Here's how the part is built. I have some questions about the finished solid (model axes, mm). Give positions to 0.01 mm unless a question says otherwise; leave off trailing zeros. Loops run counter-clockwise (first coordinate to the right, second up) from the corner with the lowest first, then second, coordinate; pieces in that order, holes last. Notation, with made-up numbers: (-17, -31.75) - (40, -31.75) arc R22 cw to (40, 3.25) - close; hole circle Ø1 at (-10, 83). An arc over 180 degrees is marked (long way). Return JSON: item names as keys, results as strings. Group by question number.
(1) If we section it at B-B (y = -24.5): Please give me the cut outline in (x, z), then the cut area to 3 significant figures.
(2) If we section it at C-C (x = 5.5): Please give me the cut outline in (y, z), then the cut area to 3 significant figures.
(3) I need wall thicknesses on probe 1 along Y at (x, z) = (22, 9); probe 2 along Y at (x, z) = (25, 9); probe 3 along X at (y, z) = (-15, 1.75). Which ranges of each line are inside material? Lowest first, please. Write a range as [from, to].
(4) For P1, Ø1.5, axis at y = -22, z = 7, coming from the +X side; P2, Ø1.5, axis at x = 22.5, z = 8.5, coming from the -Y side, each with a flat end and sliding along its axis, tell me the tip position at first contact or that it passes through.
(5) If we section it at A-A (z = 2.25): Please give me the cut outline in (x, y).
```python
from build123d import *

# Parameters (mm, degrees)
PAD_DEPTH = 10
FILLET_R  = 5


with BuildPart() as part:
    # Sketch → Pad (new body)
    with BuildSketch(Plane.XY):
        Polygon((-30, 17.320508), (-30, -17.320508), (0, -34.641016), (30, -17.320508), (30, 17.320508), (0, 34.641016), align=None)
    extrude(amount=PAD_DEPTH)

    # Fillet
    fillet_edges = [part.edges().sort_by_distance(p)[0] for p in [
        (-30, 17.320508, 5),
        (-30, -17.320508, 5),
        (0, -34.641016, 5),
        (30, -17.320508, 5),
        (30, 17.320508, 5),
        (0, 34.641016, 5),
    ]]
    fillet(fillet_edges, radius=FILLET_R)


solid = part.part
```
Values:
{
 "1": {"outline": "(-17.56, 0) - (17.56, 0) - (17.56, 10) - (-17.56, 10) - close", "area": "351 mm2"},
 "2": {"outline": "(-31.47, 0) - (31.47, 0) - (31.47, 10) - (-31.47, 10) - close", "area": "629 mm2"},
 "3": {"probe 1": "[-21.94, 21.94]", "probe 2": "[-20.21, 20.21]", "probe 3": "[-29.97, 29.97]"},
 "4": {"P1": "x = 23.19", "P2": "y = -22.08"},
 "5": {"outline": "(-30, -14.43) arc R5 ccw to (-27.5, -18.76) - (-2.5, -33.2) arc R5 ccw to (2.5, -33.2) - (27.5, -18.76) arc R5 ccw to (30, -14.43) - (30, 14.43) arc R5 ccw to (27.5, 18.76) - (2.5, 33.2) arc R5 ccw to (-2.5, 33.2) - (-27.5, 18.76) arc R5 ccw to (-30, 14.43) - close"}
}
